```python
from build123d import *

# Parameters (mm, degrees)
SKETCH1_W                    = 11.43
SKETCH1_H                    = 11.43
BOSS_EXTRUDE1_DEPTH          = 4.7625
BOSS_EXTRUDE1_DEPTH_BACK     = 1.5875
SKETCH2_W                    = 12.954
SKETCH2_H                    = 12.954
BOSS_EXTRUDE2_DEPTH          = 1.5875
SHELL1_T                     = -1
SKETCH15_R                   = 1.499997
BOSS_EXTRUDE3_DEPTH          = 6.1595
SKETCH16_W                   = 1
SKETCH16_H                   = 9.43
SKETCH16_W_2                 = 9.43
SKETCH16_H_2                 = 1
EXTRUDE_THIN1_DEPTH          = 6.1595
BOSS_EXTRUDE4_REACH          = 9.938
SKETCH17_W                   = 10.954
SKETCH17_H                   = 10.954
SKETCH17_W_2                 = 9.43
SKETCH17_H_2                 = 9.43
FILLET7_R                    = 0.508
FILLET8_R                    = 0.508
F_56_0_0465_DIAMETER_HOLE1_D = 1.1811


with BuildPart() as part:
    # Sketch1 → Boss-Extrude1 (new body, two sides)
    with BuildSketch(Plane.XY) as boss_extrude1_sk:
        Rectangle(SKETCH1_W, SKETCH1_H)
    extrude(amount=BOSS_EXTRUDE1_DEPTH)
    extrude(boss_extrude1_sk.sketch, amount=-BOSS_EXTRUDE1_DEPTH_BACK)

    # Sketch2 → Boss-Extrude2 (add)
    with BuildSketch(Plane(origin=(0, 0, -1.5875), x_dir=(-1, 0, 0), z_dir=(0, 0, -1))):
        Rectangle(SKETCH2_W, SKETCH2_H)
    extrude(amount=BOSS_EXTRUDE2_DEPTH)

    # Shell1
    shell1_openings = [part.faces().sort_by_distance(p)[0] for p in [
        (0, 0, 4.7625),
        (0, 0, -3.175),
    ]]
    offset(amount=SHELL1_T, openings=shell1_openings, kind=Kind.INTERSECTION)



with BuildPart() as body_2:
    # Sketch15 → Boss-Extrude3 (new body)
    with BuildSketch(Plane(origin=(0, 0, -3.175), x_dir=(-1, 0, 0), z_dir=(0, 0, -1))):
        Circle(SKETCH15_R)
    extrude(amount=-BOSS_EXTRUDE3_DEPTH)


with BuildPart() as part_1:
    add(part.part)

    add(body_2.part)  # Extrude-Thin1 merges body 2
    # Sketch16 → Extrude-Thin1 (add)
    with BuildSketch(Plane.XY.offset(2.9845)):
        Rectangle(SKETCH16_W, SKETCH16_H)
        Rectangle(SKETCH16_W_2, SKETCH16_H_2)
    extrude(amount=-EXTRUDE_THIN1_DEPTH)

    # Sketch17 → Boss-Extrude4 (add, up to next)
    with BuildSketch(Plane(origin=(0, 0, -3.175), x_dir=(-1, 0, 0), z_dir=(0, 0, -1)), mode=Mode.PRIVATE) as boss_extrude4_sk1:
        Rectangle(SKETCH17_W, SKETCH17_H)
        Rectangle(SKETCH17_W_2, SKETCH17_H_2, mode=Mode.SUBTRACT)
    boss_extrude4_tool1 = extrude(boss_extrude4_sk1.sketch, amount=-BOSS_EXTRUDE4_REACH, mode=Mode.PRIVATE) - part_1.part
    add(boss_extrude4_tool1.solids().sort_by_distance((0, 5.322087, -3.175))[0])

    # Fillet7
    fillet7_edges = [part_1.edges().sort_by_distance(p)[0] for p in [
        (-6.477, 6.477, -2.38125),
        (6.477, 6.477, -2.38125),
        (6.477, -6.477, -2.38125),
        (-6.477, -6.477, -2.38125),
        (5.715, -5.715, 1.5875),
        (-5.715, -5.715, 1.5875),
        (-5.715, 5.715, 1.5875),
        (5.715, 5.715, 1.5875),
    ]]
    fillet(fillet7_edges, radius=FILLET7_R)

    # Fillet8
    fillet8_edges = [part_1.edges().sort_by_distance(p)[0] for p in [
        (4.715, 0.5, -0.09525),
        (-4.715, -0.5, -0.09525),
        (1.41421038, 0.5, -0.09525),
        (1.41421038, -0.5, -0.09525),
        (4.715, -0.5, -0.09525),
        (-4.715, 0.5, -0.09525),
        (4.715, 4.715, 0.79375),
        (4.715, -4.715, 0.79375),
        (-4.715, -4.715, 0.79375),
        (-4.715, 4.715, 0.79375),
        (-0.5, 4.715, -0.09525),
        (0.5, -4.715, -0.09525),
        (-0.5, -4.715, -0.09525),
        (0.5, 4.715, -0.09525),
        (0.5, 1.41421038, -0.09525),
        (0.5, -1.41421038, -0.09525),
        (-0.5, 1.41421038, -0.09525),
        (-0.5, -1.41421038, -0.09525),
        (-1.41421038, -0.5, -0.09525),
        (-1.41421038, 0.5, -0.09525),
    ]]
    fillet(fillet8_edges, radius=FILLET8_R)

    # #56 (0.0465) Diameter Hole1 (through all)
    with Locations(Plane.XY.offset(2.9845)):
        with Locations((0, 0)):
            Hole(F_56_0_0465_DIAMETER_HOLE1_D / 2)


solid = part_1.part
```
Geometry: final body of the model. Coordinates: model frame, mm. A direction names the side the tool comes from. Coordinates: 2 decimals unless noted, no trailing zeros. Loops run counter-clockwise (first coordinate to the right, second up) from the corner with the lowest first, then second, coordinate; pieces in that order, holes last. Notation, with made-up numbers: (47.5, -4) -> (53.5, -4) arc R20 cw to (53.5, 35) -> close; hole circle Ø3 at (86.25, 8.5). An arc over 180 degrees is marked (long way). Use a Markdown table: item, result. Add a question column.
(1) Pin query (flat end, axial travel): pin 1 Ø2 at (y, z) = (4, 0.5) entering from +X (3 decimals); pin 2 Ø3 at (x, y) = (-1.5, -1) entering from +Z; pin 3 Ø1.5 at (y, z) = (-4, 0) entering from -X (3 decimals). Return the tip coordinate at first contact, or that it passes through.
(2) Mould query, pull axis Y, two halves, no side actions, for faces 1 (the flat face through (3, 0.5, 0)), 2 (the flat face through (-5, 0, 4.762)), 3 (the flat face through (0, -6.477, -2)), 4 (the flat face through (3, -0.5, 0)). Classes: pulls with the +Y half, pulls with the -Y half, needs draft (parallel to the pull), parting line crosses it, or undercut.
(3) Section query B-B, the plane x = 0. Return loops of the section in (y, z) (1 decimal), plus the area to 3 significant figures.
(4) Line query: line 1 along X through (y, z) = (3.5, 0) (3 decimals); line 2 along X through (y, z) = (3.5, 3.5) (3 decimals). Output: solid intervals per line, ascending.
(5) Section query C-C, the plane z = 3.25. Return loops of the section in (x, y) (3 decimals), plus the area to 3 significant figures.
(6) Section query A-A, the plane y = 4. Return loops of the section in (x, z) (1 decimal).
(7) Access query for faces 5 (the flat face through (0, 5.715, 2)), 6 (the flat face through (0, 6.477, -2)), 7 (the flat face through (5.715, 0, 2)), 8 (the flat face through (0, -5.715, 2)), 9 (the flat face through (0.5, -3, 0)). Directions: +Z, -Z, +X, -X, +Y, -Y. A direction counts if a zero-diameter tool reaches every point of the face in a straight line with its end or side. Return the directions, or none.
Answer:
| question | item | result |
|---|---|---|
| 1 | pin 1 | stops at x = 5.715 |
| 1 | pin 2 | stops at z = 2.98 |
| 1 | pin 3 | stops at x = -5.715 |
| 2 | face 1 | undercut |
| 2 | face 2 | needs draft |
| 2 | face 3 | pulls with the -Y half |
| 2 | face 4 | undercut |
| 3 | outline | (-6.5, -3.2) -> (-0.6, -3.2) -> (-0.6, 3) -> (-4.7, 3) -> (-4.7, 4.8) -> (-5.7, 4.8) -> (-5.7, -1.6) -> (-6.5, -1.6) -> close; (0.6, -3.2) -> (6.5, -3.2) -> (6.5, -1.6) -> (5.7, -1.6) -> (5.7, 4.8) -> (4.7, 4.8) -> (4.7, 3) -> (0.6, 3) -> close |
| 3 | area | 69.1 mm^2 |
| 4 | line 1 | x = -5.715 to -4.715, -0.5 to 0.5, 4.715 to 5.715 |
| 4 | line 2 | x = -5.715 to -4.715, 4.715 to 5.715 |
| 5 | outline | (-5.715, -5.207) arc R0.508 ccw to (-5.207, -5.715) -> (5.207, -5.715) arc R0.508 ccw to (5.715, -5.207) -> (5.715, 5.207) arc R0.508 ccw to (5.207, 5.715) -> (-5.207, 5.715) arc R0.508 ccw to (-5.715, 5.207) -> close; hole (-4.715, -4.207) arc R0.508 ccw to (-4.207, -4.715) -> (4.207, -4.715) arc R0.508 ccw to (4.715, -4.207) -> (4.715, 4.207) arc R0.508 ccw to (4.207, 4.715) -> (-4.207, 4.715) arc R0.508 ccw to (-4.715, 4.207) -> close |
| 5 | area | 41.7 mm^2 |
| 6 | outline | (-6.5, -3.2) -> (-4.7, -3.2) -> (-4.7, 4.8) -> (-5.7, 4.8) -> (-5.7, -1.6) -> (-6.5, -1.6) -> close; (-0.5, -3.2) -> (0.5, -3.2) -> (0.5, 3) -> (-0.5, 3) -> close; (4.7, -3.2) -> (6.5, -3.2) -> (6.5, -1.6) -> (5.7, -1.6) -> (5.7, 4.8) -> (4.7, 4.8) -> close |
| 7 | face 5 | +Z, +X, -X, +Y |
| 7 | face 6 | +Z, -Z, +X, -X, +Y |
| 7 | face 7 | +Z, +X, +Y, -Y |
| 7 | face 8 | +Z, +X, -X, -Y |
| 7 | face 9 | +Z, -Z |
